Part model, mm, in its own coordinate system. Face numbers are marked on the shaded views. A direction names the side the tool comes from. Round coordinates to 2 decimals unless told otherwise and drop trailing zeros. Loops run counter-clockwise (first coordinate to the right, second up) from the corner with the lowest first, then second, coordinate; pieces in that order, holes last. Notation, with made-up numbers: M 16.5,-19.75 L 61.5,-19.75 A23 ccw 61.5,4.25 Z; hole C 25,71.25 d6. An arc over 180 degrees is marked long. Put each result on its own line as item: value. Start each with the question number.
1) Slice it at C-C on z = 24.5. Give the cut face in (x, y).
2) Drop flat-ended pins along their axis: pin 1 Ø10 at (y, z) = (4, 24.5) entering from +X; pin 2 Ø1.5 at (x, z) = (16.5, 12.5) entering from +Y; pin 3 Ø7 at (y, z) = (3, 9) entering from -X; pin 4 Ø2.5 at (x, y) = (43.5, 34.5) entering from -Z. Give the stop position or say it passes through.
3) Probe line 1 along Z through (x, y) = (47, 3); line 2 along X through (y, z) = (3, 56); line 3 along X through (y, z) = (17.5, 27). List the from-to ranges inside material, lowest first.
4) Which spindle directions (+Z, -Z, +X, -X, +Y, -Y) get a long thin tool onto all of the face, cutting with end or side? Do the marked faces 1, 2, 3, 4 and 5. Say none if no direction does.
5) Slice it at A-A on z = 37. Give the cut face in (x, y), then the cut area to 3 significant figures.
6) Pull direction X, two halves, no side cores. Call the marked faces 6, 7, 8 and 9: +X half, -X half, draft (parallel to the pull), parting line (faces both ways), or undercut.
7) Slice it at B-B on x = 30.5. Give the cut face in (y, z).
8) Slice it at D-D on x = 9. Give the cut face in (y, z).
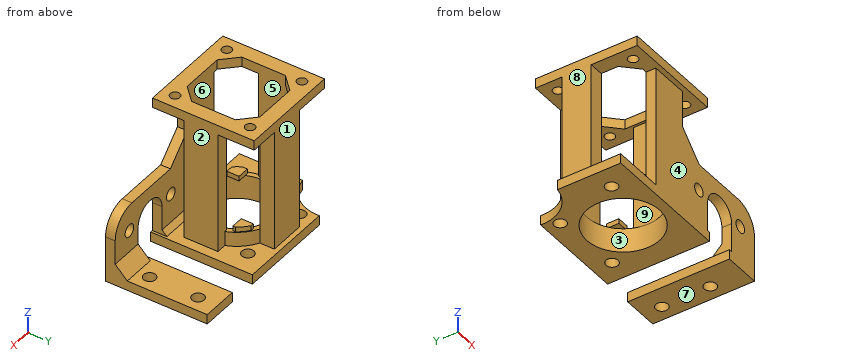
```python
from build123d import *

# Parameters (mm, degrees)
BOX009_W        = 12
BOX009_H        = 50
BOX009_DEPTH    = 10
BOX008_W        = 43
BOX008_H        = 4
BOX008_DEPTH    = 25
SKETCH006_R     = 2.5781
POCKET005_DEPTH = 4.001
FILLET_R        = 10
BOX007_W        = 5
BOX007_H        = 5
BOX007_DEPTH    = 2
SKETCH004_R     = 22
SKETCH004_R_2   = 17
POCKET003_DEPTH = 4
BOX001_W        = 15
BOX001_H        = 6
BOX001_DEPTH    = 50
BOX002_W        = 16
BOX002_H        = 4
BOX002_DEPTH    = 50
BOX004_W        = 6
BOX004_H        = 12
BOX004_DEPTH    = 50
BOX003_W        = 5
BOX003_H        = 14
BOX003_DEPTH    = 50
BOX_W           = 80
BOX_H           = 42
BOX_DEPTH       = 4
SKETCH_R        = 15
SKETCH_R_2      = 2.5
POCKET_DEPTH    = 4.001
SKETCH001_R     = 17
PAD_DEPTH       = 6
SKETCH002_R     = 15
POCKET001_DEPTH = 10.001
BOX005_W        = 42
BOX005_H        = 42
BOX005_DEPTH    = 4
SKETCH003_R     = 2
POCKET002_DEPTH = 4.001
BOX006_W        = 5
BOX006_H        = 5
BOX006_DEPTH    = 2
SKETCH005_R     = 22
SKETCH005_R_2   = 17
POCKET004_DEPTH = 4
CHAMFER_SIZE    = 5
CHAMFER001_SIZE = 2
CHAMFER002_SIZE = 10


with BuildPart() as cube008:
    # Box009 → Box009 (new body)
    with BuildSketch(Plane(origin=(53, -4, 0), x_dir=(1, 0, 0), z_dir=(0, 0, 1))):
        with Locations((6, 25)):
            Rectangle(BOX009_W, BOX009_H)
    extrude(amount=BOX009_DEPTH)


with BuildPart() as fillet_body:
    # Box008 → Box008 (new body)
    with BuildSketch(Plane(origin=(37, 0, 4), x_dir=(1, 0, 0), z_dir=(0, 0, 1))):
        with Locations((21.5, 2)):
            Rectangle(BOX008_W, BOX008_H)
    extrude(amount=BOX008_DEPTH)

    # Sketch006 → Pocket005 (cut, through all)
    with BuildSketch(Plane(origin=(37, 0, 4), x_dir=(1, 0, 0), z_dir=(0, -1, 0))):
        with Locations((34.5, 14)):
            Circle(SKETCH006_R)
        with Locations((9.753, 14)):
            Circle(SKETCH006_R)
        with BuildLine():
            ThreePointArc((29.3, 12.000026), (22.149987, 19.15), (15, 12))
            Line((15, 12), (15, 0))
            Line((15, 0), (29.3, 0))
            Line((29.3, 12.000026), (29.3, 0))
        make_face()
    extrude(amount=-POCKET005_DEPTH, mode=Mode.SUBTRACT)

    # Fillet
    fillet_edges = [fillet_body.edges().sort_by_distance(p)[0] for p in [
        (80, 2, 29),
    ]]
    fillet(fillet_edges, radius=FILLET_R)


with BuildPart() as pocket003:
    # Box007 → Box007 (new body)
    with BuildSketch(Plane(origin=(38, 27, 10), x_dir=(1, 0, 0), z_dir=(0, 0, 1))):
        with Locations((2.5, 2.5)):
            Rectangle(BOX007_W, BOX007_H)
    extrude(amount=BOX007_DEPTH)

    # Sketch004 → Pocket003 (cut)
    with BuildSketch(Plane(origin=(38, 27, 12), x_dir=(1, 0, 0), z_dir=(0, 0, 1))):
        with Locations((-9, -8.5)):
            Circle(SKETCH004_R)
        with Locations((-9, -8.5)):
            Circle(SKETCH004_R_2, mode=Mode.SUBTRACT)
    extrude(amount=-POCKET003_DEPTH, mode=Mode.SUBTRACT)


with BuildPart() as cube:
    # Box001 → Box001 (new body)
    with BuildSketch(Plane(origin=(22, 34, 4), x_dir=(1, 0, 0), z_dir=(0, 0, 1))):
        with Locations((7.5, 3)):
            Rectangle(BOX001_W, BOX001_H)
    extrude(amount=BOX001_DEPTH)


with BuildPart() as cube001:
    # Box002 → Box002 (new body)
    with BuildSketch(Plane(origin=(21, 0, 4), x_dir=(1, 0, 0), z_dir=(0, 0, 1))):
        with Locations((8, 2)):
            Rectangle(BOX002_W, BOX002_H)
    extrude(amount=BOX002_DEPTH)


with BuildPart() as cube003:
    # Box004 → Box004 (new body)
    with BuildSketch(Plane(origin=(7, 17, 4), x_dir=(1, 0, 0), z_dir=(0, 0, 1))):
        with Locations((3, 6)):
            Rectangle(BOX004_W, BOX004_H)
    extrude(amount=BOX004_DEPTH)


with BuildPart() as cube002:
    # Box003 → Box003 (new body)
    with BuildSketch(Plane(origin=(44, 11, 4), x_dir=(1, 0, 0), z_dir=(0, 0, 1))):
        with Locations((2.5, 7)):
            Rectangle(BOX003_W, BOX003_H)
    extrude(amount=BOX003_DEPTH)


with BuildPart() as fusion:
    # Box → Box (new body)
    with BuildSketch(Plane.XY):
        with Locations((40, 21)):
            Rectangle(BOX_W, BOX_H)
    extrude(amount=BOX_DEPTH)

    # Sketch → Pocket (cut, through all)
    with BuildSketch(Plane.XY.offset(4)):
        with Locations((-2, 41)):
            Circle(SKETCH_R)
        with Locations((29, 19)):
            Circle(SKETCH_R)
        with Locations((9, 10)):
            Circle(SKETCH_R_2)
        with Locations((16, 36)):
            Circle(SKETCH_R_2)
        with Locations((44.1, 34)):
            Circle(SKETCH_R_2)
        with Locations((73.9, 34)):
            Circle(SKETCH_R_2)
        with Locations((73.9, 14)):
            Circle(SKETCH_R_2)
    extrude(amount=-POCKET_DEPTH, mode=Mode.SUBTRACT)

    # Sketch001 → Pad (new body)
    with BuildSketch(Plane.XY.offset(4)):
        with Locations((29, 19)):
            Circle(SKETCH001_R)
    extrude(amount=PAD_DEPTH)

    # Sketch002 → Pocket001 (cut, through all)
    with BuildSketch(Plane.XY.offset(10)):
        with Locations((29, 19)):
            Circle(SKETCH002_R)
    extrude(amount=-POCKET001_DEPTH, mode=Mode.SUBTRACT)

    # Fusion: union Cube, Cube001, Cube003, Cube002
    add(cube.part)
    add(cube001.part)
    add(cube003.part)
    add(cube002.part)


with BuildPart() as fusion001:
    # Box005 → Box005 (new body)
    with BuildSketch(Plane(origin=(7, -2, 54), x_dir=(1, 0, 0), z_dir=(0, 0, 1))):
        with Locations((21, 21)):
            Rectangle(BOX005_W, BOX005_H)
    extrude(amount=BOX005_DEPTH)

    # Sketch003 → Pocket002 (cut, through all)
    with BuildSketch(Plane(origin=(7, -2, 58), x_dir=(1, 0, 0), z_dir=(0, 0, 1))):
        with Locations((5.5, 36.5)):
            Circle(SKETCH003_R)
        with Locations((36.5, 36.5)):
            Circle(SKETCH003_R)
        with Locations((5.5, 5.5)):
            Circle(SKETCH003_R)
        with Locations((36.5, 5.5)):
            Circle(SKETCH003_R)
        Polygon((6, 30), (6, 12), (12, 6), (30, 6), (36, 12), (36, 30), (30, 36), (12, 36), align=None)
    extrude(amount=-POCKET002_DEPTH, mode=Mode.SUBTRACT)

    # Fusion001: union Fusion
    add(fusion.part)


with BuildPart() as chamfer002:
    # Box006 → Box006 (new body)
    with BuildSketch(Plane(origin=(14, 8, 10), x_dir=(1, 0, 0), z_dir=(0, 0, 1))):
        with Locations((2.5, 2.5)):
            Rectangle(BOX006_W, BOX006_H)
    extrude(amount=BOX006_DEPTH)

    # Sketch005 → Pocket004 (cut)
    with BuildSketch(Plane(origin=(14, 8, 12), x_dir=(1, 0, 0), z_dir=(0, 0, 1))):
        with Locations((15, 11)):
            Circle(SKETCH005_R)
        with Locations((15, 11)):
            Circle(SKETCH005_R_2, mode=Mode.SUBTRACT)
    extrude(amount=-POCKET004_DEPTH, mode=Mode.SUBTRACT)

    # Fusion002: union Pocket003, Fusion001
    add(pocket003.part)
    add(fusion001.part)

    # Fusion003: union Fillet body
    add(fillet_body.part)

    # Chamfer
    chamfer_edges = [chamfer002.edges().sort_by_distance(p)[0] for p in [
        (73.15, 4, 4),
    ]]
    chamfer(chamfer_edges, length=CHAMFER_SIZE)

    # Chamfer001
    chamfer001_edges = [chamfer002.edges().sort_by_distance(p)[0] for p in [
        (44.5, 4, 4),
    ]]
    chamfer(chamfer001_edges, length=CHAMFER001_SIZE)

    # Cut: cut Cube008
    add(cube008.part, mode=Mode.SUBTRACT)

    # Chamfer002
    chamfer002_edges = [chamfer002.edges().sort_by_distance(p)[0] for p in [
        (37, 2, 29),
    ]]
    chamfer(chamfer002_edges, length=CHAMFER002_SIZE)


solid = chamfer002.part
```
Recorded:
1. outline: M 7,17 L 13,17 L 13,29 L 7,29 Z; M 21,0 L 78.35,0 L 78.35,4 L 21,4 Z; M 22,34 L 37,34 L 37,40 L 22,40 Z; M 44,11 L 49,11 L 49,25 L 44,25 Z
2. pin 1: stops at x = 79.99
2. pin 2: stops at y = 13
2. pin 3: stops at x = 17.48
2. pin 4: passes through
3. line 1: z = 0 to 15.43, 20.57 to 29, 54 to 58
3. line 2: x = 7 to 10.56, 14.44 to 41.56, 45.44 to 49
3. line 3: x = 7 to 13, 44 to 49
4. face 1: +Z, +X, -X, +Y
4. face 2: +Z, +X, +Y
4. face 3: -Z
4. face 4: -Z, +X, -X, -Y
4. face 5: none
5. outline: M 7,17 L 13,17 L 13,29 L 7,29 Z; M 21,0 L 39,0 L 39,4 L 21,4 Z; M 22,34 L 37,34 L 37,40 L 22,40 Z; M 44,11 L 49,11 L 49,25 L 44,25 Z
5. area: 304 mm2
6. face 6: undercut
6. face 7: draft
6. face 8: -X half
6. face 9: undercut
7. outline: M -2,54 L 0,54 L 0,0 L 4.08,0 L 4.08,10 L 4,10 L 4,58 L -2,58 Z; M 33.92,0 L 42,0 L 42,4 L 40,4 L 40,58 L 34,58 L 34,10 L 33.92,10 Z
8. outline: M -2,54 L 17,54 L 17,4 L 12.5,4 L 12.5,0 L 30.8,0 L 30.8,4 L 29,4 L 29,54 L 40,54 L 40,58 L -2,58 Z; M 0,0 L 7.5,0 L 7.5,4 L 0,4 Z
